Verification items for the finished model (mm, model axes). A direction names the side the tool comes from. Give positions to 0.01 mm unless a question says otherwise; leave off trailing zeros. Order: outer loops, then holes, each group sorted by start corner. A loop starts at its lowest first (then second) coordinate and runs counter-clockwise, first axis right, second up. Notation, with made-up numbers: M 87.25,-30.75 L 91.25,-30.75 A31 ccw 91.25,-0.75 Z; hole C -37.5,10 d4. An arc over 180 degrees is marked long. Answer as a JSON object with one key per item and string values.
```python
from build123d import *

# Parameters (mm, degrees)
BOSS_EXTRUDE1_DEPTH = 100
BOSS_EXTRUDE2_DEPTH = 50
SKETCH5_W           = 30
SKETCH5_H           = 45
CUT_EXTRUDE1_DEPTH  = 20


with BuildPart() as part:
    # Sketch3 → Boss-Extrude1 (new body)
    with BuildSketch(Plane(origin=(0, 0, 0), x_dir=(1, 0, 0), z_dir=(0, 1, 0))):
        with BuildLine():
            Line((-125, 0), (-125, 100))
            Line((-125, 100), (-100, 100))
            Line((-100, 100), (-100, 70))
            Line((-100, 70), (100, 70))
            Line((100, 70), (100, 100))
            Line((100, 100), (125, 100))
            Line((125, 100), (125, 0))
            ThreePointArc((125, 0), (0, -125), (-125, 0))
        make_face()
    extrude(amount=BOSS_EXTRUDE1_DEPTH)

    # Sketch4 → Boss-Extrude2 (add)
    with BuildSketch(Plane(origin=(0, 100, 0), x_dir=(1, 0, 0), z_dir=(0, 1, 0))):
        with BuildLine():
            Line((-100, 100), (100, 100))
            Line((100, 100), (125, 100))
            Line((125, 100), (125, 0))
            ThreePointArc((125, 0), (0, -125), (-125, 0))
            Line((-125, 0), (-125, 100))
            Line((-125, 100), (-100, 100))
        make_face()
    extrude(amount=BOSS_EXTRUDE2_DEPTH)

    # Sketch5 → Cut-Extrude1 (cut)
    with BuildSketch(Plane.XZ):
        with Locations((-98, 0)):
            Rectangle(SKETCH5_W, SKETCH5_H)
        with Locations((98, 0)):
            Rectangle(SKETCH5_W, SKETCH5_H)
    extrude(amount=-CUT_EXTRUDE1_DEPTH, mode=Mode.SUBTRACT)


solid = part.part
```
Q1. Section check A-A on z = -73. Record the cut outline in (x, y), then the cut area to 3 significant figures.
Resolved:
{"outline": "M -125,0 L -100,0 L -100,100 L 100,100 L 100,0 L 125,0 L 125,150 L -125,150 Z", "area": "17,500 mm²"}
Q2. Section check D-D on x = -41. Record the cut outline in (y, z), then the cut area to 3 significant figures.
Resolved:
{"outline": "M 0,-70 L 100,-70 L 100,-100 L 150,-100 L 150,118.08 L 0,118.08 Z", "area": "29,700 mm²"}
Q3. Gauge pin test, flat ends, axial feed: pin 1 Ø16 at (x, y) = (-91.5, 5.5) entering from +Z; pin 2 Ø6 at (x, y) = (94, 10) entering from -Z; pin 3 Ø1.5 at (x, y) = (-57, 100.5) entering from +Z. Record the tip position at first contact, or that the pin passes through.
Resolved:
{"pin 1": "stops at z = 93.02", "pin 2": "stops at z = -70", "pin 3": "stops at z = 111.63"}
Q4. Section check C-C on z = 16.5. Record the cut outline in (x, y), then the cut area to 3 significant figures.
Resolved:
{"outline": "M -123.91,0 L -113,0 L -113,20 L -83,20 L -83,0 L 83,0 L 83,20 L 113,20 L 113,0 L 123.91,0 L 123.91,150 L -123.91,150 Z", "area": "36,000 mm²"}
Q5. Section check B-B on x = 0. Record the cut outline in (y, z), then the cut area to 4 significant figures.
Resolved:
{"outline": "M 0,-70 L 100,-70 L 100,-100 L 150,-100 L 150,125 L 0,125 Z", "area": "30,750 mm²"}
Q6. Tool access check on faces 1 (the face through (-125, 74, -49)), 2 (the face through (-1, 49, -70)), 3 (the face through (98, 10, -22.5)). Record the directions out of +Z, -Z, +X, -X, +Y, -Y that give a thin tool (end or side, any length) a straight path to the whole face; none if there is none.
Resolved:
{"face 1": "+Z, -Z, -X, +Y, -Y", "face 2": "-Z, -Y", "face 3": "-Y"}
Q7. Material ranges on L1, parallel to Z at x = -1.5, y = 15; L2, parallel to X at y = 97, z = -75.5; L3, parallel to Y at x = 93.5, z = 14.5, recorded low to high.
Resolved:
{"L1": "z = -70 to 124.99", "L2": "x = -125 to -100, 100 to 125", "L3": "y = 20 to 150"}
Q8. Release check for a two-part mould opening along X. For faces 4 (the face through (-98, 20, 0)), 5 (the face through (2, 0, 11)), 6 (the face through (2.75, 73.95, 124.97)) record: +X half, -X half, draft (parallel to the pull), parting line (faces both ways), or undercut.
Resolved:
{"face 4": "undercut", "face 5": "draft", "face 6": "parting line"}
